For this review, take the finished solid that the model builds, in its own axes (mm). A direction names the side the tool comes from. Coordinates: 2 decimals unless noted, no trailing zeros. Write each loop counter-clockwise with the first axis right and the second up, starting at its lowest first coordinate (ties: lowest second). Pieces come first, ordered by that corner, then holes. Notation, with made-up numbers: (39, -22) -> (87, -22) arc R13 ccw to (87, -8) -> close; hole circle Ø2 at (-9, 88.25). An arc over 180 degrees is marked (long way). One line per item, written item: value. Start each with the question number.
1) Machinability: for faces 1 (the flat face through (0, 0, -38.5)), 2 (the flat face through (0, 1.5, -34)), 3 (the cylindrical face through (10, 0, -18)), 4 (the flat face through (0, 0, 32.8)), 5 (the cylindrical face through (-2.579, -1.978, 31.786)), which of the approach directions +Z, -Z, +X, -X, +Y, -Y give a long, thin tool a straight path to every point of the face, cutting with its end or side? Answer none if there is none.
2) Mouldability with a two-part tool opening along X and no side actions: class faces 6 (the cylindrical face through (-11.923, 3.755, -13.318)), 7 (the flat face through (-2.44, 2.44, 30.8)), 8 (the cylindrical face through (0.423, 11.722, -24.535)), 9 (the flat face through (0, 9, -9)) as released by +X, released by -X, zero draft, split by the parting line, or undercut.
3) For probe 1 along Y at (x, z) = (0, -17.5); probe 2 along Y at (x, z) = (0, -23.1); probe 3 along Z at (x, y) = (-2.25, 0.75), list the stretches that pass through material, from the lowest coordinate up. Write a range as from..to.
4) Add section B-B (z = 28). State the section outline as (x, y) points, and give its area (3 significant figures).
5) For pin 1 Ø2 at (x, z) = (0.5, -33) entering from +Y; pin 2 Ø12 at (x, z) = (-9, -29) entering from +Y; pin 3 Ø4 at (x, y) = (8.5, 0) entering from -Z, all flat-tipped, find the tip position at first contact; note any pin that passes through.
6) Add section A-A (z = -15.5). State the section outline as (x, y) points, and give its area (3 significant figures).
from build123d import *

# Parameters (mm, degrees)
SKETCH_1_R          = 12.2
EXTRUDE_1_DEPTH     = 30.8
SKETCH_2_R          = 3.25
EXTRUDE_2_DEPTH     = 2
FILLET_1_R          = 2.5
SKETCH_3_R          = 12.5
EXTRUDE_3_DEPTH     = 27
SKETCH_4_R          = 3.5
EXTRUDE_4_DEPTH     = 2.5
SKETCH_5_R          = 2
EXTRUDE_5_DEPTH     = 9
CUT_EXTRUDE_START   = -8
CUT_EXTRUDE_1_DEPTH = 8
SKETCH_7_R          = 1.5
CUT_EXTRUDE_2_DEPTH = 18
FILLET_2_R          = 0.5
SKETCH_8_R          = 3.25
CUT_EXTRUDE_3_DEPTH = 5


with BuildPart() as part:
    # ｽｹｯﾁ1 → ﾎﾞｽ - 押し出し1 (new body)
    with BuildSketch(Plane.XY):
        with Locations(Location((0, 0, 0), (0, 0, 180))):
            Circle(SKETCH_1_R)
    extrude(amount=EXTRUDE_1_DEPTH)

    # ｽｹｯﾁ2 → ﾎﾞｽ - 押し出し2 (add)
    with BuildSketch(Plane.XY.offset(30.8)):
        Circle(SKETCH_2_R)
    extrude(amount=EXTRUDE_2_DEPTH)

    # ﾌｨﾚｯﾄ1
    fillet_1_edges = [part.edges().sort_by_distance(p)[0] for p in [
        (12.2, 0, 0),
    ]]
    fillet(fillet_1_edges, radius=FILLET_1_R)

    # ｽｹｯﾁ3 → ﾎﾞｽ - 押し出し3 (add)
    with BuildSketch(Plane(origin=(0, 0, 0), x_dir=(-1, 0, 0), z_dir=(0, 0, -1))):
        Circle(SKETCH_3_R)
    extrude(amount=EXTRUDE_3_DEPTH)

    # ｽｹｯﾁ4 → ﾎﾞｽ - 押し出し4 (add)
    with BuildSketch(Plane(origin=(0, 0, -27), x_dir=(-1, 0, 0), z_dir=(0, 0, -1))):
        Circle(SKETCH_4_R)
    extrude(amount=EXTRUDE_4_DEPTH)

    # ｽｹｯﾁ5 → ﾎﾞｽ - 押し出し5 (add)
    with BuildSketch(Plane(origin=(0, 0, -29.5), x_dir=(-1, 0, 0), z_dir=(0, 0, -1))):
        Circle(SKETCH_5_R)
    extrude(amount=EXTRUDE_5_DEPTH)

    # ｽｹｯﾁ6 → ｶｯﾄ - 押し出し1 (cut)
    with BuildSketch(Plane(origin=(0, 0, -38.5), x_dir=(-1, 0, 0), z_dir=(0, 0, -1)).offset(CUT_EXTRUDE_START)):
        with BuildLine():
            Line((-1.322875656, 1.5), (1.322875656, 1.5))
            ThreePointArc((1.322875656, 1.5), (0, 2), (-1.322875656, 1.5))
        make_face()
    extrude(amount=CUT_EXTRUDE_1_DEPTH, mode=Mode.SUBTRACT)

    # ｽｹｯﾁ7 → ｶｯﾄ - 押し出し2 (cut)
    with BuildSketch(Plane(origin=(0, 0, -27), x_dir=(-1, 0, 0), z_dir=(0, 0, -1))):
        with Locations((0, 8.5)):
            Circle(SKETCH_7_R)
        with Locations((8.5, 0)):
            Circle(SKETCH_7_R)
        with Locations((0, -8.5)):
            Circle(SKETCH_7_R)
        with Locations((-8.5, 0)):
            Circle(SKETCH_7_R)
    extrude(amount=-CUT_EXTRUDE_2_DEPTH, mode=Mode.SUBTRACT)

    # ﾌｨﾚｯﾄ2
    fillet_2_edges = [part.edges().sort_by_distance(p)[0] for p in [
        (12.5, 0, 0),
        (12.5, 0, -27),
        (12.2, 0, 30.8),
    ]]
    fillet(fillet_2_edges, radius=FILLET_2_R)

    # ｽｹｯﾁ8 → ｶｯﾄ - 押し出し3 (cut)
    with BuildSketch(Plane(origin=(0, 0, -27), x_dir=(-1, 0, 0), z_dir=(0, 0, -1))):
        with Locations((0, 8.5)):
            Circle(SKETCH_8_R)
        with Locations((0, -8.5)):
            Circle(SKETCH_8_R)
    extrude(amount=-CUT_EXTRUDE_3_DEPTH, mode=Mode.SUBTRACT)


solid = part.part
Numbers:
1. face 1: -Z, +X, -X, +Y, -Y
1. face 2: -Z, +X, -X, +Y
1. face 3: -Z
1. face 4: +Z, +X, -X, +Y, -Y
1. face 5: +Z
2. face 6: split by the parting line
2. face 7: zero draft
2. face 8: undercut
2. face 9: undercut
3. probe 1: -12.5..-10, -7..7, 10..12.5
3. probe 2: -12.5..-11.75, -5.25..5.25, 11.75..12.5
3. probe 3: -29.5..32.8
4. outline: circle Ø24.4 at (0, 0)
4. area: 468 mm²
5. pin 1: y = 1.5
5. pin 2: y = 11.99
5. pin 3: z = -27
6. outline: circle Ø25 at (0, 0); hole circle Ø3 at (-8.5, 0); hole circle Ø3 at (0, -8.5); hole circle Ø3 at (0, 8.5); hole circle Ø3 at (8.5, 0)
6. area: 463 mm²
